```python
from build123d import *

# Parameters (mm, degrees)
SKETCH1_R               = 1.6
BOSS_EXTRUDE1_DEPTH     = 2
SKETCH2_R               = 0.5
BOSS_EXTRUDE2_DEPTH     = 2
SKETCH3_R               = 1.6
BOSS_EXTRUDE3_DEPTH     = 4
SKETCH4_R               = 5.618069601
SKETCH4_R_2             = 1.5
SKETCH4_R_3             = 9.019483561
CUT_EXTRUDE1_DEPTH      = 20
CUT_EXTRUDE2_DEPTH      = 10
CUT_EXTRUDE2_DEPTH_BACK = 10
SKETCH6_W               = 4
SKETCH6_H               = 1
SKETCH6_R               = 0.5
BOSS_EXTRUDE5_DEPTH     = 2
SKETCH7_R               = 9
SKETCH7_R_2             = 5
BOSS_EXTRUDE6_DEPTH     = 2
SKETCH8_R               = 5
CUT_EXTRUDE3_DEPTH      = 10


with BuildPart() as part:
    # Sketch1 → Boss-Extrude1 (new body)
    with BuildSketch(Plane(origin=(0, 0, 0), x_dir=(1, 0, 0), z_dir=(0, 1, 0))):
        with BuildLine():
            Line((0, 3), (70, 3))
            ThreePointArc((70, 3), (73, 0), (70, -3))
            Line((70, -3), (0, -3))
            ThreePointArc((0, -3), (-3, 0), (0, 3))
        make_face()
        Circle(SKETCH1_R, mode=Mode.SUBTRACT)
        with Locations((70, 0)):
            Circle(SKETCH1_R, mode=Mode.SUBTRACT)
        with Locations((35, 0)):
            Circle(SKETCH1_R, mode=Mode.SUBTRACT)
    extrude(amount=BOSS_EXTRUDE1_DEPTH)

    # Sketch2 → Boss-Extrude2 (add)
    with BuildSketch(Plane(origin=(0, 2, 0), x_dir=(1, 0, 0), z_dir=(0, 1, 0))):
        with BuildLine():
            Line((37, -3), (33, -3))
            Line((33, -3), (33, -14))
            ThreePointArc((33, -14), (35, -16), (37, -14))
            Line((37, -14), (37, -3))
        make_face()
        with Locations((35, -11.5)):
            Circle(SKETCH2_R, mode=Mode.SUBTRACT)
        with Locations((35, -14)):
            Circle(SKETCH2_R, mode=Mode.SUBTRACT)
        with Locations((35, -9.5)):
            Circle(SKETCH2_R, mode=Mode.SUBTRACT)
        with BuildLine():
            Line((33, 14), (33, 3))
            Line((33, 3), (37, 3))
            Line((37, 3), (37, 14))
            ThreePointArc((37, 14), (35, 16), (33, 14))
        make_face()
        with Locations((35, 9.5)):
            Circle(SKETCH2_R, mode=Mode.SUBTRACT)
        with Locations((35, 14)):
            Circle(SKETCH2_R, mode=Mode.SUBTRACT)
        with Locations((35, 11.5)):
            Circle(SKETCH2_R, mode=Mode.SUBTRACT)
    extrude(amount=-BOSS_EXTRUDE2_DEPTH)

    # Sketch3 → Boss-Extrude3 (add)
    with BuildSketch(Plane(origin=(0, 0, 0), x_dir=(-1, 0, 0), z_dir=(0, -1, 0))):
        with Locations((-70, 0)):
            Circle(SKETCH3_R)
        Circle(SKETCH3_R)
    extrude(amount=-BOSS_EXTRUDE3_DEPTH)

    # Sketch4 → Cut-Extrude1 (cut)
    with BuildSketch(Plane(origin=(0, 2, 0), x_dir=(1, 0, 0), z_dir=(0, 1, 0))):
        with Locations((70, 0)):
            Circle(SKETCH4_R)
        with Locations((70, 0)):
            Circle(SKETCH4_R_2, mode=Mode.SUBTRACT)
        Circle(SKETCH4_R_3)
        Circle(SKETCH4_R_2, mode=Mode.SUBTRACT)
    extrude(amount=CUT_EXTRUDE1_DEPTH, mode=Mode.SUBTRACT)

    # Sketch5 → Cut-Extrude2 (cut, two sides)
    with BuildSketch(Plane(origin=(0, 2, 0), x_dir=(1, 0, 0), z_dir=(0, 1, 0))) as cut_extrude2_sk:
        with BuildLine():
            Line((55, 1.6), (70, 1.6))
            ThreePointArc((70, 1.6), (71.6, 0), (70, -1.6))
            Line((70, -1.6), (55, -1.6))
            ThreePointArc((55, -1.6), (53.4, 0), (55, 1.6))
        make_face()
        with BuildLine():
            Line((0, -1.6), (15, -1.6))
            ThreePointArc((15, -1.6), (16.6, 0), (15, 1.6))
            Line((15, 1.6), (0, 1.6))
            ThreePointArc((0, 1.6), (-1.6, 0), (0, -1.6))
        make_face()
    extrude(amount=CUT_EXTRUDE2_DEPTH, mode=Mode.SUBTRACT)
    extrude(cut_extrude2_sk.sketch, amount=-CUT_EXTRUDE2_DEPTH_BACK, mode=Mode.SUBTRACT)

    # Sketch6 → Boss-Extrude5 (add)
    with BuildSketch(Plane(origin=(0, 2, 0), x_dir=(1, 0, 0), z_dir=(0, 1, 0))):
        with Locations((35, 3.5)):
            Rectangle(SKETCH6_W, SKETCH6_H)
        with BuildLine():
            Line((33, 4), (0, 4))
            ThreePointArc((0, 4), (-4, 0), (0, -4))
            Line((0, -4), (33, -4))
            Line((33, -4), (33, -3))
            Line((33, -3), (0, -3))
            ThreePointArc((0, -3), (-3, 0), (0, 3))
            Line((0, 3), (33, 3))
            Line((33, 3), (33, 4))
        make_face()
        with BuildLine():
            Line((70, 4), (37, 4))
            Line((37, 4), (37, 3))
            Line((37, 3), (70, 3))
            ThreePointArc((70, 3), (73, 0), (70, -3))
            Line((70, -3), (37, -3))
            Line((37, -3), (37, -4))
            Line((37, -4), (70, -4))
            ThreePointArc((70, -4), (74, 0), (70, 4))
        make_face()
        with Locations((35, -3.5)):
            Rectangle(SKETCH6_W, SKETCH6_H)
        with BuildLine():
            Line((33, 14), (33, 4))
            Line((33, 4), (37, 4))
            Line((37, 4), (37, 14))
            ThreePointArc((37, 14), (35, 16), (33, 14))
        make_face()
        with Locations((35, 9.5)):
            Circle(SKETCH6_R, mode=Mode.SUBTRACT)
        with Locations((35, 11.5)):
            Circle(SKETCH6_R, mode=Mode.SUBTRACT)
        with Locations((35, 14)):
            Circle(SKETCH6_R, mode=Mode.SUBTRACT)
    extrude(amount=-BOSS_EXTRUDE5_DEPTH)

    # Sketch7 → Boss-Extrude6 (add)
    with BuildSketch(Plane(origin=(0, 2, 0), x_dir=(1, 0, 0), z_dir=(0, 1, 0))):
        with Locations((35, 0)):
            Circle(SKETCH7_R)
        with Locations((35, 0)):
            Circle(SKETCH7_R_2, mode=Mode.SUBTRACT)
    extrude(amount=-BOSS_EXTRUDE6_DEPTH)

    # Sketch8 → Cut-Extrude3 (cut)
    with BuildSketch(Plane(origin=(0, 2, 0), x_dir=(1, 0, 0), z_dir=(0, 1, 0))):
        with Locations((35, 0)):
            Circle(SKETCH8_R)
    extrude(amount=-CUT_EXTRUDE3_DEPTH, mode=Mode.SUBTRACT)


solid = part.part
```
Geometry: final body of the model. Coordinates: model frame, mm. A direction names the side the tool comes from. Give positions to 0.01 mm unless a question says otherwise; leave off trailing zeros. Loops run counter-clockwise (first coordinate to the right, second up) from the corner with the lowest first, then second, coordinate; pieces in that order, holes last. Notation, with made-up numbers: (-4, 69.25) -> (44, 69.25) arc R15 cw to (44, 84.25) -> close; hole circle Ø7 at (-7, -25). An arc over 180 degrees is marked (long way). Use one line per item in the form item = value.
Item 1: Section query B-B on x = 59.5. Output: boundary loops of the cut face in (y, z).
A:
outline = (0, -4) -> (2, -4) -> (2, -1.6) -> (0, -1.6) -> close; (0, 1.6) -> (2, 1.6) -> (2, 4) -> (0, 4) -> close
Item 2: Line query: probe 1 along Z at (x, y) = (66, 1.95); probe 2 along X at (y, z) = (0.55, 9.5); probe 3 along Z at (x, y) = (52.5, 1.35). Output: solid intervals per line, ascending.
A:
probe_1 = -4 to -1.6, 1.6 to 4
probe_2 = 33 to 34.5, 35.5 to 37
probe_3 = -4 to 4
Item 3: Section query C-C on y = 1.2. Give the number of separate pieces and of enclosed holes in the cut face, and give its area (3 significant figures).
A:
separate_pieces = 1
enclosed_holes = 9
area = 583 mm^2
Item 4: Section query A-A on z = 0. Output: boundary loops of the cut face in (x, y), and give its area (3 significant figures).
A:
outline = (-4, 0) -> (-1.6, 0) -> (-1.6, 2) -> (-4, 2) -> close; (16.6, 0) -> (30, 0) -> (30, 2) -> (16.6, 2) -> close; (40, 0) -> (53.4, 0) -> (53.4, 2) -> (40, 2) -> close; (71.6, 0) -> (74, 0) -> (74, 2) -> (71.6, 2) -> close
area = 63.2 mm^2
Item 5: Pin query (flat end, axial travel): P1, Ø1, axis at y = 1, z = -12.5, coming from the -X side; P2, Ø0.6, axis at x = 63, y = 1.5, coming from the +Z side; P3, Ø0.6, axis at x = 10.5, y = 1.5, coming from the -Z side; P4, Ø8, axis at x = 35, z = 0, coming from the -Y side. Return the tip coordinate at first contact, or that it passes through.
A:
P1 = 33
P2 = 4
P3 = -4
P4 = through
Item 6: Access query for faces 1 (the face through (14, 1, -4)), 2 (the face through (71.6, 1, 0)), 3 (the face through (-4, 1, 0)), 4 (the face through (33, 1, 11)), 5 (the face through (56, 1, 4)). Directions: +Z, -Z, +X, -X, +Y, -Y. A direction counts if a zero-diameter tool reaches every point of the face in a straight line with its end or side. Return the directions, or none.
A:
face_1 = -Z, -X, +Y, -Y
face_2 = +Y, -Y
face_3 = -X, +Y, -Y
face_4 = +Z, -X, +Y, -Y
face_5 = +Z, +X, +Y, -Y
Item 7: Section query D-D on x = 41.5. Output: boundary loops of the cut face in (y, z).
A:
outline = (0, -6.22) -> (2, -6.22) -> (2, 6.22) -> (0, 6.22) -> close
Item 8: Draft query along Z for faces 6 (the face through (33, 1, -11)), 7 (the face through (30, 1, 0)), 8 (the face through (40.525, 1.014, 7.105)). Return one class per face: pulls with the +Z half, pulls with the -Z half, needs draft (parallel to the pull), parting line crosses it, or undercut.
A:
face_6 = needs draft
face_7 = undercut
face_8 = pulls with the +Z half
